Read the model definition and answer for the solid it produces. Units are mm, in the model's axes. Face numbers are marked on the shaded views. A direction names the side the tool comes from. Coordinates: 2 decimals unless noted, no trailing zeros. Write each loop counter-clockwise with the first axis right and the second up, starting at its lowest first coordinate (ties: lowest second). Pieces come first, ordered by that corner, then holes. Notation, with made-up numbers: M 74.25,16.25 L 82.25,16.25 A17 ccw 82.25,45.25 Z; hole C -3.5,23 d5. An arc over 180 degrees is marked long. Write item = value, one per line.
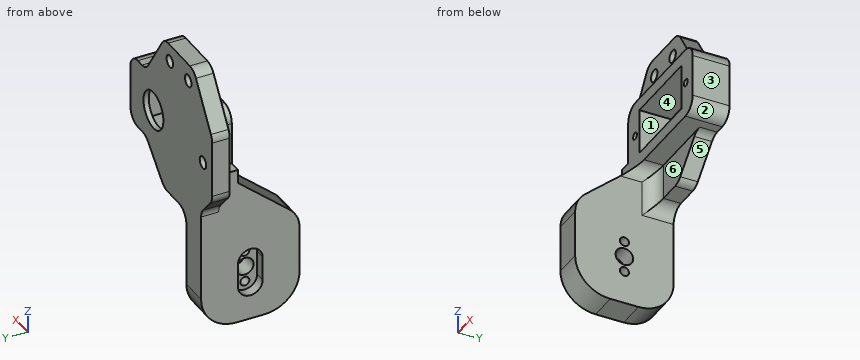
from build123d import *

# Parameters (mm, degrees)
BOSS_EXTRUDE1_DEPTH            = 38.4
SKETCH2_W                      = 38.4
SKETCH2_H                      = 15
BOSS_EXTRUDE2_DEPTH            = 5.5
SKETCH3_W                      = 38.4
SKETCH3_H                      = 23
BOSS_EXTRUDE3_DEPTH            = 27
SKETCH8_W                      = 38.4
SKETCH8_H                      = 5.5
BOSS_EXTRUDE4_DEPTH            = 20
CUT_EXTRUDE1_DEPTH             = 30.4
SKETCH10_W                     = 30.4
SKETCH10_H                     = 5.5
CUT_EXTRUDE2_DEPTH             = 32
BOSS_EXTRUDE5_DEPTH            = 5
CUT_EXTRUDE3_REACH             = 89.653
SKETCH17_W                     = 16.045256013
SKETCH17_H                     = 5.5
CUT_EXTRUDE4_DEPTH             = 94.189913617
CUT_EXTRUDE5_DEPTH             = 5.5
CUT_EXTRUDE6_DEPTH             = 3
SKETCH34_W                     = 23
SKETCH34_H                     = 13
CUT_EXTRUDE7_DEPTH             = 9
F_3_5_3_5_DIAMETER_HOLE1_D     = 3.5
F_10_8_10_8_DIAMETER_HOLE1_D   = 10.8
F_5_0_5_DIAMETER_HOLE1_D       = 5
F_5_0_5_DIAMETER_HOLE1_DEPTH   = 35.4
F_2_6_2_6_DIAMETER_HOLE1_D     = 2.6
F_2_6_2_6_DIAMETER_HOLE1_DEPTH = 14
F_2_0_2_DIAMETER_HOLE1_D       = 2
F_2_0_2_DIAMETER_HOLE1_DEPTH   = 7
FILLET1_R                      = 4
FILLET2_R                      = 8
FILLET3_R                      = 10


with BuildPart() as part:
    # Sketch1 → Boss-Extrude1 (new body)
    with BuildSketch(Plane(origin=(44.4, 0, 0), x_dir=(0, 0, -1), z_dir=(1, 0, 0))):
        Polygon((50, -5.5), (35, -5.5), (50, -23), align=None)
    extrude(amount=-BOSS_EXTRUDE1_DEPTH)

    # Sketch2 → Boss-Extrude2 (add)
    with BuildSketch(Plane(origin=(0, -5.5, 0), x_dir=(-1, 0, 0), z_dir=(0, 1, 0))):
        with Locations((-25.2, -42.5)):
            Rectangle(SKETCH2_W, SKETCH2_H)
    extrude(amount=BOSS_EXTRUDE2_DEPTH)

    # Sketch3 → Boss-Extrude3 (add)
    with BuildSketch(Plane(origin=(0, 0, -50), x_dir=(-1, 0, 0), z_dir=(0, 0, -1))):
        with Locations((-25.2, -11.5)):
            Rectangle(SKETCH3_W, SKETCH3_H)
    extrude(amount=BOSS_EXTRUDE3_DEPTH)

    # Sketch8 → Boss-Extrude4 (add)
    with BuildSketch(Plane.XY.offset(-35)):
        with Locations((25.2, -2.75)):
            Rectangle(SKETCH8_W, SKETCH8_H)
    extrude(amount=BOSS_EXTRUDE4_DEPTH)

    # Sketch9 → Cut-Extrude1 (cut)
    with BuildSketch(Plane(origin=(44.4, 0, 0), x_dir=(0, 0, -1), z_dir=(1, 0, 0))):
        Polygon((77, -23), (77, -5.5), (35, -5.5), (50, -23), align=None)
    extrude(amount=-CUT_EXTRUDE1_DEPTH, mode=Mode.SUBTRACT)

    # Sketch10 → Cut-Extrude2 (cut)
    with BuildSketch(Plane(origin=(0, 0, -77), x_dir=(-1, 0, 0), z_dir=(0, 0, -1))):
        with Locations((-29.2, -2.75)):
            Rectangle(SKETCH10_W, SKETCH10_H)
    extrude(amount=-CUT_EXTRUDE2_DEPTH, mode=Mode.SUBTRACT)

    # Sketch11 → Boss-Extrude5 (add)
    with BuildSketch(Plane(origin=(0, 0, 0), x_dir=(-1, 0, 0), z_dir=(0, 1, 0))):
        Polygon((-10, 0), (0, -15), (0, -33.819660113), (-6, -40.527864045), (-6, -77), (-14, -77), (-14, -45), (-44.4, -45), (-44.4, -15), (-36, -15), (-26, 0), align=None)
    extrude(amount=BOSS_EXTRUDE5_DEPTH)

    # Sketch17 → Cut-Extrude3 (cut, up to next)
    with BuildSketch(Plane(origin=(9.4, 0, 0), x_dir=(0, 0, -1), z_dir=(1, 0, 0)), mode=Mode.PRIVATE) as cut_extrude3_sk1:
        with Locations((23.022628007, -2.75)):
            Rectangle(SKETCH17_W, SKETCH17_H)
    cut_extrude3_tool1 = extrude(cut_extrude3_sk1.sketch, amount=-CUT_EXTRUDE3_REACH, mode=Mode.PRIVATE) & part.part
    add(cut_extrude3_tool1.solids().sort_by_distance((9.4, -2.75, -23.022628))[0], mode=Mode.SUBTRACT)

    # Sketch24 → Cut-Extrude4 (cut, through all)
    with BuildSketch(Plane(origin=(0, 5, 0), x_dir=(-1, 0, 0), z_dir=(0, 1, 0))):
        Polygon((-36, -35), (-44.4, -35), (-44.4, -45), (-26, -45), align=None)
    extrude(amount=-CUT_EXTRUDE4_DEPTH, mode=Mode.SUBTRACT)

    # Sketch25 → Cut-Extrude5 (cut)
    with BuildSketch(Plane.XZ.offset(5.5)):
        Polygon((36, -35), (14, -35), (14, -45), (26, -45), align=None)
    extrude(amount=-CUT_EXTRUDE5_DEPTH, mode=Mode.SUBTRACT)

    # Sketch33 → Cut-Extrude6 (cut)
    with BuildSketch(Plane.ZY.offset(-6)):
        with BuildLine():
            Line((-66.5, -12.5), (-59.5, -12.5))
            ThreePointArc((-59.5, -12.5), (-56, -9), (-59.5, -5.5))
            Line((-59.5, -5.5), (-66.5, -5.5))
            ThreePointArc((-66.5, -5.5), (-70, -9), (-66.5, -12.5))
        make_face()
    extrude(amount=-CUT_EXTRUDE6_DEPTH, mode=Mode.SUBTRACT)

    # Sketch34 → Cut-Extrude7 (cut)
    with BuildSketch(Plane.XZ.offset(5.5)):
        with Locations((26.9, -25)):
            Rectangle(SKETCH34_W, SKETCH34_H)
    extrude(amount=-CUT_EXTRUDE7_DEPTH, mode=Mode.SUBTRACT)

    # Ø3.5 (3.5) Diameter Hole1 (through all)
    with Locations(Plane(origin=(0, 0, 0), x_dir=(-1, 0, 0), z_dir=(0, -1, 0))):
        with Locations((-5, 25), (-13, 5), (-23, 5)):
            Hole(F_3_5_3_5_DIAMETER_HOLE1_D / 2)

    # Ø10.8 (10.8) Diameter Hole1 (through all)
    with Locations(Plane(origin=(0, 3.5, 0), x_dir=(-1, 0, 0), z_dir=(0, -1, 0))):
        with Locations((-31.9, 25)):
            Hole(F_10_8_10_8_DIAMETER_HOLE1_D / 2)

    # Ø5.0 (5) Diameter Hole1
    with Locations(Plane.ZY.offset(-9)):
        with Locations((-63, -9)):
            Hole(F_5_0_5_DIAMETER_HOLE1_D / 2, depth=F_5_0_5_DIAMETER_HOLE1_DEPTH)

    # Ø2.6 (2.6) Diameter Hole1
    with Locations(Plane(origin=(14, 0, 0), x_dir=(0, 0, -1), z_dir=(1, 0, 0))):
        with Locations((58.5, -9), (67.5, -9)):
            Hole(F_2_6_2_6_DIAMETER_HOLE1_D / 2, depth=F_2_6_2_6_DIAMETER_HOLE1_DEPTH)

    # Ø2.0 (2) Diameter Hole1
    with Locations(Plane(origin=(0, -5.5, 0), x_dir=(-1, 0, 0), z_dir=(0, -1, 0))):
        with Locations((-13.1, 25), (-40.7, 25)):
            Hole(F_2_0_2_DIAMETER_HOLE1_D / 2, depth=F_2_0_2_DIAMETER_HOLE1_DEPTH)

    # Fillet1
    fillet1_edges = [part.edges().sort_by_distance(p)[0] for p in [
        (9.4, -2.75, -15),
        (44.4, -0.25, -35),
        (36, 2.5, -35),
        (26, 2.5, -45),
        (14, 2.5, -45),
        (14, 0, -40),
        (14, -2.75, -35),
        (44.4, -0.25, -15),
        (10, 2.5, 0),
        (26, 2.5, 0),
        (36, 2.5, -15),
        (6, 2.5, -40.527864045),
        (0, 2.5, -33.819660113),
        (0, 2.5, -15),
    ]]
    fillet(fillet1_edges, radius=FILLET1_R)

    # Fillet2
    fillet2_edges = [part.edges().sort_by_distance(p)[0] for p in [
        (10, -23, -50),
    ]]
    fillet(fillet2_edges, radius=FILLET2_R)

    # Fillet3
    fillet3_edges = [part.edges().sort_by_distance(p)[0] for p in [
        (10, -23, -77),
        (10, 5, -77),
    ]]
    fillet(fillet3_edges, radius=FILLET3_R)


solid = part.part
Item 1: Consider line 1 along X through (y, z) = (1.15, -25); line 2 along Z through (x, y) = (24, -0.25); line 3 along X through (y, z) = (-3.5, -25). Determine where each line is inside the solid, lowest interval first. Write a range as from..to.
Worked answers:
line_1 = 0..3.25, 6.75..12.1, 14.1..15.4, 38.4..39.7, 41.7..44.4
line_2 = -35..-31.5, -18.5..-15
line_3 = 9.4..12.1, 14.1..15.4, 38.4..39.7, 41.7..44.4
Item 2: Which of the six approach directions +Z, -Z, +X, -X, +Y, -Y give full straight-line access (tool end or side, diameter ignored) to the marked faces 4, 5 and 6?
Worked answers:
face_4 = -Y
face_5 = -Z, +X, +Y, -Y
face_6 = -Z, +X, -Y
Item 3: Find section D-D (z = -5). Determine the outline of the cut face in (x, y).
Worked answers:
outline = M 6.67,0 L 11.25,0 L 11.25,5 L 6.67,5 Z; M 14.75,0 L 21.25,0 L 21.25,5 L 14.75,5 Z; M 24.75,0 L 29.33,0 L 29.33,5 L 24.75,5 Z
Item 4: Find section B-B (z = -63). Determine the outline of the cut face in (x, y).
Worked answers:
outline = M 6,-23 L 14,-23 L 14,-11.5 L 9,-11.5 L 9,-12.5 L 6,-12.5 Z; M 6,-5.5 L 9,-5.5 L 9,-6.5 L 14,-6.5 L 14,5 L 6,5 Z
Item 5: Flat-ended cylindrical pins translate along their axes: pin 1 (5.5 mm diameter, centred on x = 21, y = 3, fed in from -Z); pin 2 (8.5 mm diameter, centred on x = 32, y = 1.5, fed in from -Z); pin 3 (10 mm diameter, centred on y = -4, z = -39.5, fed in from +X). Find the tip coordinate at first contact, or state that the pin passes through.
Worked answers:
pin_1 = -45
pin_2 = -43.25
pin_3 = 42.34
Item 6: Find section C-C (y = -9). Determine the outline of the cut face in (x, z), and give its area (3 significant figures).
Worked answers:
outline = M 6,-77 L 14,-77 L 14,-68.8 L 9,-68.8 L 9,-70 L 6,-70 Z; M 6,-56 L 9,-56 L 9,-57.2 L 14,-57.2 L 14,-39 A4 cw 14.13,-38 L 6,-38 Z; M 9,-66.2 L 14,-66.2 L 14,-65.5 L 9,-65.5 Z; M 9,-60.5 L 14,-60.5 L 14,-59.8 L 9,-59.8 Z
area = 219 mm²
Item 7: Find section A-A (x = 31.9). Determine the outline of the cut face in (y, z).
Worked answers:
outline = M -5.5,-35 L 0,-35 L 0,-39.1 L 5,-39.1 L 5,-30.4 L 3.5,-30.4 L 3.5,-31.5 L -5.5,-31.5 Z; M -5.5,-18.5 L 3.5,-18.5 L 3.5,-19.6 L 5,-19.6 L 5,-8.85 L 0,-8.85 L 0,-15 L -5.5,-15 Z
Item 8: For a pull along Z with two mould halves and no side action, classify the marked faces 1, 2 and 3 as released by +Z, released by -Z, zero draft, split by the parting line, or undercut.
Worked answers:
face_1 = undercut
face_2 = released by -Z
face_3 = zero draft
